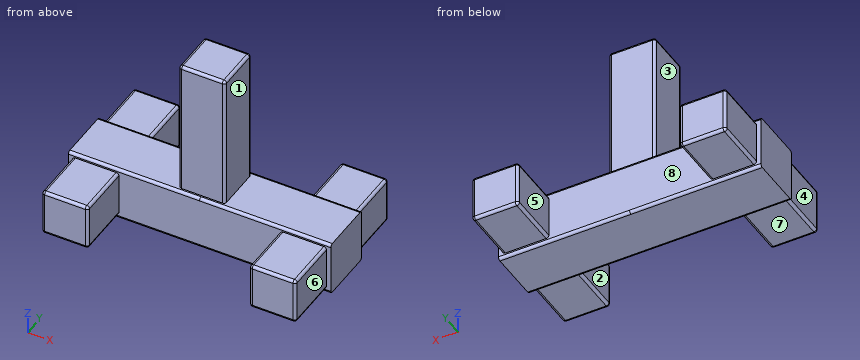
```python
from build123d import *

# Parameters (mm, degrees)
SKETCH1_W            = 20
SKETCH1_H            = 20
SKETCH1_W_2          = 16.9
SKETCH1_H_2          = 16.9
SKETCH1_W_3          = 28
BOSS_EXTRUDE3_DEPTH  = 20
BOSS_EXTRUDE4_START  = -20
SKETCH1_6_W          = 16.9
SKETCH1_6_H          = 16.9
BOSS_EXTRUDE4_DEPTH  = 60
FILLET2_R            = 1
FILLET2_OF_MIRROR1_R = 1
SKETCH3_W            = 16.9
SKETCH3_H            = 16.9
BOSS_EXTRUDE5_DEPTH  = 50
FILLET3_R            = 1


with BuildPart() as part:
    # Sketch1 → Boss-Extrude3 (new body)
    with BuildSketch(Plane(origin=(0, 0, 0), x_dir=(1, 0, 0), z_dir=(0, 1, 0))):
        with Locations((-38, 0)):
            Rectangle(SKETCH1_W, SKETCH1_H)
        with Locations((-38, 0)):
            Rectangle(SKETCH1_W_2, SKETCH1_H_2, mode=Mode.SUBTRACT)
        with Locations((-38, 0)):
            Rectangle(SKETCH1_W_2, SKETCH1_H_2)
        with Locations((-14, 0)):
            Rectangle(SKETCH1_W_3, SKETCH1_H)
    boss_extrude3 = extrude(amount=BOSS_EXTRUDE3_DEPTH)

    # Sketch1_6 → Boss-Extrude4 (add)
    with BuildSketch(Plane(origin=(0, 0, 0), x_dir=(1, 0, 0), z_dir=(0, 1, 0)).offset(BOSS_EXTRUDE4_START)):
        with Locations((-38, 0)):
            Rectangle(SKETCH1_6_W, SKETCH1_6_H)
    boss_extrude4 = extrude(amount=BOSS_EXTRUDE4_DEPTH)

    # Fillet2
    fillet2_edges = [part.edges().sort_by_distance(p)[0] for p in [
        (-24, 20, 10),
        (-29.55, -10, 8.45),
        (-46.45, -10, 8.45),
        (-24, 20, -10),
        (-38, -20, -8.45),
        (-46.45, -10, -8.45),
        (-29.55, -20, 0),
        (-29.55, -10, -8.45),
        (-29.55, 30, 8.45),
        (-38, 40, 8.45),
        (-46.45, 30, 8.45),
        (-46.45, 40, 0),
        (-46.45, 30, -8.45),
        (-29.55, 30, -8.45),
        (-38, -20, 8.45),
        (-46.45, -20, 0),
        (-29.55, 40, 0),
        (-38, 40, -8.45),
        (-24, 0, -10),
        (-24, 0, 10),
    ]]
    fillet(fillet2_edges, radius=FILLET2_R)

    # Mirror1: Boss-Extrude3, Boss-Extrude4 across plane
    add(boss_extrude3.mirror(Plane(origin=(0, 20, 0), x_dir=(0, 0, 1), z_dir=(1, 0, 0))))
    add(boss_extrude4.mirror(Plane(origin=(0, 20, 0), x_dir=(0, 0, 1), z_dir=(1, 0, 0))))

    # Fillet2 of Mirror1
    fillet2_of_mirror1_edges = [part.edges().sort_by_distance(p)[0] for p in [
        (24, 20, 10),
        (29.55, -10, 8.45),
        (46.45, -10, 8.45),
        (24, 20, -10),
        (38, -20, -8.45),
        (46.45, -10, -8.45),
        (29.55, -20, 0),
        (29.55, -10, -8.45),
        (29.55, 30, 8.45),
        (38, 40, 8.45),
        (46.45, 30, 8.45),
        (46.45, 40, 0),
        (46.45, 30, -8.45),
        (29.55, 30, -8.45),
        (38, -20, 8.45),
        (46.45, -20, 0),
        (29.55, 40, 0),
        (38, 40, -8.45),
        (24, 0, -10),
        (24, 0, 10),
    ]]
    fillet(fillet2_of_mirror1_edges, radius=FILLET2_OF_MIRROR1_R)

    # Sketch3 → Boss-Extrude5 (add)
    with BuildSketch(Plane.XY.offset(10)):
        with Locations((0, 10)):
            Rectangle(SKETCH3_W, SKETCH3_H)
    extrude(amount=BOSS_EXTRUDE5_DEPTH)

    # Fillet3
    fillet3_edges = [part.edges().sort_by_distance(p)[0] for p in [
        (-8.45, 10, 60),
        (-8.45, 18.45, 35),
        (-8.45, 1.55, 35),
        (8.45, 1.55, 35),
        (0, 18.45, 60),
        (8.45, 18.45, 35),
        (0, 1.55, 60),
        (8.45, 10, 60),
    ]]
    fillet(fillet3_edges, radius=FILLET3_R)


solid = part.part
```
Can you work these out from the model? Positions are in its coordinate system, mm. Face numbers are marked on the shaded views. A direction names the side the tool comes from. Give positions to 0.01 mm unless a question says otherwise; leave off trailing zeros. Write each loop counter-clockwise with the first axis right and the second up, starting at its lowest first coordinate (ties: lowest second). Pieces come first, ordered by that corner, then holes. Notation, with made-up numbers: (55, 63.5) - (76, 63.5) arc R23 cw to (76, 100.5) - close; hole circle Ø5 at (35.25, 62.5). An arc over 180 degrees is marked (long way). Write item = value, one per line. Start each with the question number.
1. Imagine slicing it at A-A (y = 5.5). Please give me the cut outline in (x, z), and give its area (3 significant figures).
2. Imagine slicing it at B-B (y = -2). Please give me the cut outline in (x, z).
3. Imagine slicing it at D-D (x = -39.5). Please give me the cut outline in (y, z), and give its area (3 significant figures).
4. Imagine slicing it at C-C (z = 26.5). Please give me the cut outline in (x, y).
5. Thinking about a two-plate mould opening in X: for the marked faces 6, 7 and 8, which applies, released by +X, released by -X, zero draft, split by the parting line, or undercut?
6. On a 3-axis mill with a long thin cutter (end or side, diameter ignored), from which of +Z, -Z, +X, -X, +Y, -Y can I reach the whole of each face in a straight line? I mean the marked faces 1, 2, 3, 4 and 5. Say none if no direction works.
7. Please list where these lines run through material, in increasing order: line 1 (Y direction, x = -23, z = 9); line 2 (Z direction, x = 43, y = 30); line 3 (X direction, y = -5, z = -7).
8. For pin 1 (16.5 mm diameter, centred on x = 35, y = 27, fed in from -Z); pin 2 (7.5 mm diameter, centred on x = -40.5, y = -8.5, fed in from -Z); pin 3 (12 mm diameter, centred on x = -9, z = 35, fed in from -Y); pin 4 (12 mm diameter, centred on x = 40.5, y = -13, fed in from +Z), each with a flat end and sliding along its axis, tell me the tip position at first contact or that it passes through.
Worked answers:
q1.outline = (-48, -10) - (48, -10) - (48, 10) - (8.45, 10) - (8.45, 59) arc R1 ccw to (7.45, 60) - (-7.45, 60) arc R1 ccw to (-8.45, 59) - (-8.45, 10) - (-48, 10) - close
q1.area = 2,760 mm2
q2.outline = (-46.45, -7.45) arc R1 ccw to (-45.45, -8.45) - (-30.55, -8.45) arc R1 ccw to (-29.55, -7.45) - (-29.55, 7.45) arc R1 ccw to (-30.55, 8.45) - (-45.45, 8.45) arc R1 ccw to (-46.45, 7.45) - close; (29.55, -7.45) arc R1 ccw to (30.55, -8.45) - (45.45, -8.45) arc R1 ccw to (46.45, -7.45) - (46.45, 7.45) arc R1 ccw to (45.45, 8.45) - (30.55, 8.45) arc R1 ccw to (29.55, 7.45) - close
q3.outline = (-20, -7.45) arc R1 ccw to (-19, -8.45) - (0, -8.45) - (0, -9) arc R1 ccw to (1, -10) - (19, -10) arc R1 ccw to (20, -9) - (20, -8.45) - (39, -8.45) arc R1 ccw to (40, -7.45) - (40, 7.45) arc R1 ccw to (39, 8.45) - (20, 8.45) - (20, 9) arc R1 ccw to (19, 10) - (1, 10) arc R1 ccw to (0, 9) - (0, 8.45) - (-19, 8.45) arc R1 ccw to (-20, 7.45) - close
q3.area = 1,070 mm2
q4.outline = (-8.45, 2.55) arc R1 ccw to (-7.45, 1.55) - (7.45, 1.55) arc R1 ccw to (8.45, 2.55) - (8.45, 17.45) arc R1 ccw to (7.45, 18.45) - (-7.45, 18.45) arc R1 ccw to (-8.45, 17.45) - close
q5.face_6 = released by +X
q5.face_7 = zero draft
q5.face_8 = undercut
q6.face_1 = +Z, +X, +Y, -Y
q6.face_2 = +Z, -Z, -Y
q6.face_3 = +Z, -X, +Y, -Y
q6.face_4 = +Z, -Z, -X, -Y
q6.face_5 = +Z, -Z, +Y
q7.line_1 = 0 to 20
q7.line_2 = -8.45 to 8.45
q7.line_3 = -46.45 to -29.55, 29.55 to 46.45
q8.pin_1 = -10
q8.pin_2 = -8.45
q8.pin_3 = 1.55
q8.pin_4 = 8.45
